Verification items for the finished model (mm, model axes). Coordinates: 2 decimals unless noted, no trailing zeros. Loops run counter-clockwise (first coordinate to the right, second up) from the corner with the lowest first, then second, coordinate; pieces in that order, holes last.
Q1. Sectioned sample at A-A (z = -1). Enter the section's corners in (x, y), then the cut area to 4 significant figures.
Q2. Material ranges on probe 1 along Y at (x, z) = (0.25, 13); probe 2 along Z at (x, y) = (1.4, 7.5); probe 3 along Z at (x, y) = (0.7, -5.5), recorded low to high.
Q3. Sectioned sample at B-B (x = 0.3). Count the separate pieces of the cut face and the enclosed holes in it, then the cut area to 3 significant figures.
Q4. Go/stop test with flat-tipped pins: P1, Ø0.8, axis at x = 1, y = -20.5, coming from the +Z side; P2, Ø0.8, axis at x = 1, z = -39, coming from the +Y side; P3, Ø0.8, axis at x = 0.5, y = -24.5, coming from the -Z side. Record where each tip stops, or that it passes through.
```python
from build123d import *

# Parameters (mm, degrees)
F0_R     = 1
F0_R_2   = 1.5
F1_DEPTH = 1.5


# Not quite as in the source:
# - ends of sketch curves that miss each other by under 0.0002 mm in the source are joined


with BuildPart() as f1:
    # F0 (on Right) → F1 (new body)
    with BuildSketch(Plane.YZ):
        with BuildLine():
            Line((-21.996098, -27.31987), (-21.996098, -45.812627))
            Line((-21.996098, -45.812627), (-17.621845, -50.438265))
            ThreePointArc((-17.621845, -50.438265), (-15.2556042555, -51.8397305124), (-12.5061720552, -51.7778968223))
            ThreePointArc((-12.5061720552, -51.7778968223), (3.5454625901, -40.4951161641), (9.9951640259, -21.9652090006))
            ThreePointArc((9.9951640259, -21.9652090006), (10.2757378346, -20.9894720288), (10.9992601785, -20.2772223111))
            ThreePointArc((10.9992601785, -20.2772223111), (12.0039002073, -18.545177798), (11.0039019167, -16.8104491443))
            ThreePointArc((11.0039019167, -16.8104491443), (10.2718512165, -16.0783980417), (10.003902, -15.078398))
            Line((10.003902, -15.078398), (10.003902, 4.921602))
            ThreePointArc((10.003902, 4.921602), (10.2718512165, 5.9216020417), (11.0039020833, 6.6536528557))
            ThreePointArc((11.0039020833, 6.6536528557), (12.003902, 8.3856934558), (11.0039201798, 10.1177443114))
            ThreePointArc((11.0039201798, 10.1177443114), (10.269458941, 10.8540026976), (10.0039615857, 11.8594979972))
            ThreePointArc((10.0039615857, 11.8594979972), (10.3891645141, 13.7598432984), (11.4683680941, 15.3707479059))
            Line((11.4683680941, 15.3707479059), (21.774273, 25.676653))
            ThreePointArc((21.774273, 25.676653), (24.7317604297, 31.0578388491), (24.3439893135, 37.185932113))
            ThreePointArc((24.3439893135, 37.185932113), (21.7900626838, 42.4607965791), (18.1940737554, 47.088495765))
            ThreePointArc((18.1940737554, 47.088495765), (10.2755723108, 51.5882270472), (1.1845109874, 51.0379080347))
            Line((1.1845109874, 51.0379080347), (-5.280894, 48.684693))
            ThreePointArc((-5.280894, 48.684693), (-10.7177919764, 45.6790606822), (-14.9701240908, 41.1501140619))
            ThreePointArc((-14.9701240908, 41.1501140619), (-18.4726000988, 37.9865656192), (-23.0359049993, 36.7817319627))
            ThreePointArc((-23.0359049993, 36.7817319627), (-24.4243161193, 36.1821969282), (-24.996098, 34.782128))
            Line((-24.996098, 34.782128), (-24.996098, 32.779751))
            Line((-24.996098, 32.779751), (-22.996098, 32.779751))
            ThreePointArc((-22.996098, 32.779751), (-22.496098, 33.279751), (-21.996098, 32.779751))
            Line((-21.996098, 32.779751), (-21.996098, 17.279751))
            Line((-21.996098, 17.279751), (-15.831989, 17.279751))
            ThreePointArc((-15.831989, 17.279751), (-15.570936575, 17.2626407174), (-15.3143508308, 17.2116026314))
            Line((-15.3143508308, 17.2116026314), (-1.366688, 13.474338))
            ThreePointArc((-1.366688, 13.474338), (-1.0994211963, 13.2957555405), (-0.996098, 12.991375))
            Line((-0.996098, 12.991375), (-0.996098, -22.132359))
            ThreePointArc((-0.996098, -22.132359), (-1.0994211963, -22.4367395405), (-1.3666880537, -22.6153217996))
            Line((-1.3666880537, -22.6153217996), (-18.669968, -27.251722))
            ThreePointArc((-18.669968, -27.251722), (-18.9265537033, -27.3027597343), (-19.187606, -27.31987))
            Line((-19.187606, -27.31987), (-21.996098, -27.31987))
        make_face()
        with Locations((-19.496098, -35.419491)):
            Circle(F0_R, mode=Mode.SUBTRACT)
        with BuildLine():
            ThreePointArc((-17.7460980692, -36.3877369617), (-17.496098, -35.419491), (-17.7460980692, -34.4512450383))
            ThreePointArc((-17.7460980692, -34.4512450383), (-17.9325896552, -33.9829990692), (-17.996098, -33.482999))
            Line((-17.996098, -33.482999), (-17.996098, -32.478968))
            ThreePointArc((-17.996098, -32.478968), (-17.3761580188, -30.6526837103), (-15.7725551288, -29.5811905194))
            Line((-15.7725551288, -29.5811905194), (-11.424682, -28.416182))
            ThreePointArc((-11.424682, -28.416182), (-8.6270574238, -28.4772261134), (-6.3003638496, -30.0318728738))
            Line((-6.3003638496, -30.0318728738), (-1.723529, -35.486332))
            ThreePointArc((-1.723529, -35.486332), (-0.5624401991, -38.9949163794), (-2.1282627813, -42.3425262325))
            ThreePointArc((-2.1282627813, -42.3425262325), (-6.3573337492, -45.6393399924), (-11.1210981684, -48.1011625838))
            ThreePointArc((-11.1210981684, -48.1011625838), (-15.7911829634, -47.6118199936), (-17.996098, -43.466039))
            Line((-17.996098, -43.466039), (-17.996098, -37.355982))
            ThreePointArc((-17.996098, -37.355982), (-17.9325897646, -36.8559823544), (-17.7460980692, -36.3877369617))
        make_face(mode=Mode.SUBTRACT)
        with Locations((2.550308, -37.579716)):
            Circle(F0_R_2, mode=Mode.SUBTRACT)
        with BuildLine():
            Line((0.417191, -31.973043), (-2.175306, -28.883425))
            ThreePointArc((-2.175306, -28.883425), (-2.5506520894, -26.9964379968), (-1.1608561692, -25.6659973686))
            Line((-1.1608561692, -25.6659973686), (2.673734, -24.638522))
            ThreePointArc((2.673734, -24.638522), (4.5680584745, -25.1196037387), (5.1476802368, -26.9861360503))
            ThreePointArc((5.1476802368, -26.9861360503), (4.5711819336, -29.2325622712), (3.8091151123, -31.4230040444))
            ThreePointArc((3.8091151123, -31.4230040444), (2.2694207433, -32.6616792107), (0.417191, -31.973043))
        make_face(mode=Mode.SUBTRACT)
        with BuildLine():
            Line((2.753902, -15.078398), (2.753902, 4.921602))
            ThreePointArc((2.753902, 4.921602), (4.503902, 6.671602), (6.253902, 4.921602))
            Line((6.253902, 4.921602), (6.253902, -15.078398))
            ThreePointArc((6.253902, -15.078398), (4.503902, -16.828398), (2.753902, -15.078398))
        make_face(mode=Mode.SUBTRACT)
        with Locations((-19.496098, 25.279751)):
            Circle(F0_R, mode=Mode.SUBTRACT)
        with BuildLine():
            Line((-6.767723, 18.027369), (-14.425805, 20.079346))
            ThreePointArc((-14.425805, 20.079346), (-15.9042612839, 22.1361274193), (-14.1808899041, 23.992515303))
            Line((-14.1808899041, 23.992515303), (-6.577551, 25.039093))
            ThreePointArc((-6.577551, 25.039093), (-4.8203932786, 24.3980923464), (-4.3615548361, 22.5848209601))
            ThreePointArc((-4.3615548361, 22.5848209601), (-4.477484693, 21.5402984379), (-4.3247299968, 20.5005230009))
            ThreePointArc((-4.3247299968, 20.5005230009), (-4.8272219648, 18.553710138), (-6.767723, 18.027369))
        make_face(mode=Mode.SUBTRACT)
        with BuildLine():
            ThreePointArc((-14.5567540245, 28.1495958796), (-16.7346535441, 29.9536300539), (-16.4449966717, 32.7667927786))
            Line((-16.4449966717, 32.7667927786), (-12.351599, 38.835505))
            ThreePointArc((-12.351599, 38.835505), (-12.1477989547, 39.1318667137), (-11.9387027549, 39.4245158215))
            ThreePointArc((-11.9387027549, 39.4245158215), (-10.058959181, 40.2298668034), (-8.4541402996, 38.9623558853))
            Line((-8.4541402996, 38.9623558853), (-8.060642, 37.934613))
            ThreePointArc((-8.060642, 37.934613), (-7.9933516406, 36.7140017623), (-8.6490128126, 35.6822417749))
            ThreePointArc((-8.6490128126, 35.6822417749), (-10.9344787533, 33.0050906706), (-12.1959899918, 29.7188949984))
            ThreePointArc((-12.1959899918, 29.7188949984), (-13.050327583, 28.4437625647), (-14.5567540245, 28.1495958796))
        make_face(mode=Mode.SUBTRACT)
        with BuildLine():
            ThreePointArc((-8.3564720989, 28.2540276311), (-9.0243989567, 28.7665460217), (-9.1342894359, 29.6012468489))
            ThreePointArc((-9.1342894359, 29.6012468489), (-7.221617113, 32.914093113), (-3.9087709469, 34.8267658017))
            ThreePointArc((-3.9087709469, 34.8267658017), (-3.0740700217, 34.7168759567), (-2.5615515641, 34.0489488489))
            Line((-2.5615515641, 34.0489488489), (-2.486494, 33.76883))
            ThreePointArc((-2.486494, 33.76883), (-2.5963839786, 32.9341291338), (-3.2643109011, 32.4216106311))
            ThreePointArc((-3.2643109011, 32.4216106311), (-5.4609207948, 31.1533976608), (-6.7291343423, 28.9567880917))
            ThreePointArc((-6.7291343423, 28.9567880917), (-7.2416529097, 28.288861108), (-8.0763538489, 28.1789705641))
            Line((-8.0763538489, 28.1789705641), (-8.3564720989, 28.2540276311))
        make_face(mode=Mode.SUBTRACT)
        with Locations((-1.996098, 27.688574)):
            Circle(F0_R_2, mode=Mode.SUBTRACT)
        with Locations((-8.121383, 43.686669)):
            Circle(F0_R, mode=Mode.SUBTRACT)
        with BuildLine():
            Line((-1.430644, 21.3282), (-1.505702, 21.608318))
            ThreePointArc((-1.505702, 21.608318), (-1.3958117152, 22.4430193965), (-0.7278839158, 22.9555376859))
            ThreePointArc((-0.7278839158, 22.9555376859), (1.4687256608, 24.2237512052), (2.7369386593, 26.4203610913))
            ThreePointArc((2.7369386593, 26.4203610913), (3.2494571338, 27.0882880214), (4.0841580989, 27.1981783689))
            Line((4.0841580989, 27.1981783689), (4.364277, 27.123121))
            ThreePointArc((4.364277, 27.123121), (5.0322040214, 26.6106028662), (5.1420943689, 25.7759019011))
            ThreePointArc((5.1420943689, 25.7759019011), (3.229421546, 22.46305532), (-0.0834248031, 20.5503822653))
            ThreePointArc((-0.0834248031, 20.5503822653), (-0.9181258662, 20.6602729786), (-1.430644, 21.3282))
        make_face(mode=Mode.SUBTRACT)
        with Locations((7.503902, 13.146944)):
            Circle(F0_R, mode=Mode.SUBTRACT)
        with BuildLine():
            ThreePointArc((8.2610496287, 25.9707480622), (8.8217830592, 27.0570250546), (9.9099700271, 27.6140428345))
            Line((9.9099700271, 27.6140428345), (13.098357, 28.136825))
            ThreePointArc((13.098357, 28.136825), (15.2015024129, 27.0760034199), (14.8361780624, 24.7489659376))
            Line((14.8361780624, 24.7489659376), (10.150334, 20.063122))
            ThreePointArc((10.150334, 20.063122), (7.5177667465, 19.8912658497), (7.0051173965, 22.4791483493))
            ThreePointArc((7.0051173965, 22.4791483493), (7.7900633915, 24.1684823506), (8.2610496287, 25.9707480622))
        make_face(mode=Mode.SUBTRACT)
        with BuildLine():
            Line((-2.49442, 45.955934), (2.394616, 47.735397))
            ThreePointArc((2.394616, 47.735397), (3.4373252946, 48.0640337253), (4.5047620376, 48.3003037863))
            ThreePointArc((4.5047620376, 48.3003037863), (7.5818252173, 46.9139330558), (7.422211849, 43.5427511135))
            Line((7.422211849, 43.5427511135), (3.45896, 38.27169))
            ThreePointArc((3.45896, 38.27169), (2.4608377023, 37.5658778413), (1.2383930198, 37.5728080606))
            ThreePointArc((1.2383930198, 37.5728080606), (-0.5497351994, 37.9875076656), (-2.3829199888, 38.0813777001))
            ThreePointArc((-2.3829199888, 38.0813777001), (-3.5599861465, 38.4114308125), (-4.3250867004, 39.3648671147))
            Line((-4.3250867004, 39.3648671147), (-4.861895, 40.766909))
            ThreePointArc((-4.861895, 40.766909), (-4.7654691919, 43.8575037621), (-2.49442, 45.955934))
        make_face(mode=Mode.SUBTRACT)
        with BuildLine():
            ThreePointArc((11.859796151, 42.7887138865), (14.1961631415, 43.985186443), (16.5795798456, 42.8854218737))
            ThreePointArc((16.5795798456, 42.8854218737), (18.1256065821, 40.7697438525), (19.4317694803, 38.4981297378))
            ThreePointArc((19.4317694803, 38.4981297378), (19.4257656197, 34.8830903624), (16.5076749457, 32.7492453311))
            Line((16.5076749457, 32.7492453311), (7.512064, 31.274283))
            ThreePointArc((7.512064, 31.274283), (5.4774784003, 32.2122847196), (5.5899054074, 34.4498604456))
            Line((5.5899054074, 34.4498604456), (11.859796151, 42.7887138865))
        make_face(mode=Mode.SUBTRACT)
        with Locations((21.958067, 30.811764)):
            Circle(F0_R, mode=Mode.SUBTRACT)
    extrude(amount=F1_DEPTH)


solid = f1.part
```
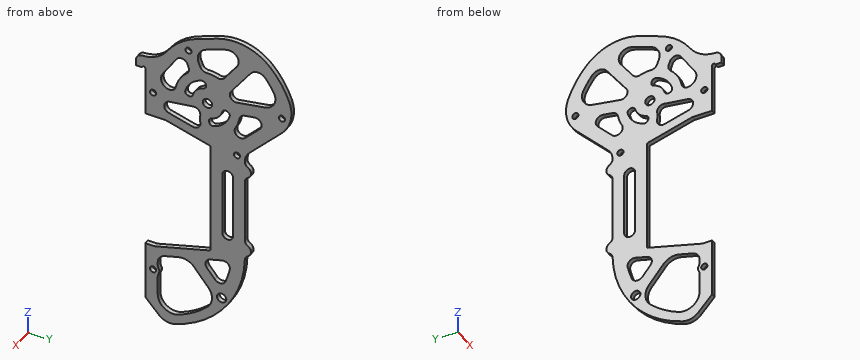
Geometry check:
1. outline: (0, -1) - (1.5, -1) - (1.5, 2.75) - (0, 2.75) - close; (0, 6.25) - (1.5, 6.25) - (1.5, 10) - (0, 10) - close
1. area: 11.25 mm2
2. probe 1: y = -1 to 6.51, 8.49 to 10.14
2. probe 2: z = -33.63 to 12.15, 14.15 to 19.91, 23.45 to 31.27, 36.99 to 43.65, 47.04 to 51.98
2. probe 3: z = -48.64 to -45.07, -30.99 to -23.72, 14.58 to 18.11, 24.89 to 31.11, 34.2 to 48.6
3. separate pieces: 1
3. enclosed holes: 17
3. area: 1,630 mm2
4. P1: stops at z = 37.28
4. P2: stops at y = 4.87
4. P3: stops at z = 32.78
